Here's how the part is built. I have some questions about the finished solid (model axes, mm). Face numbers are marked on the shaded views. Round coordinates to 2 decimals unless told otherwise and drop trailing zeros. Loops run counter-clockwise (first coordinate to the right, second up) from the corner with the lowest first, then second, coordinate; pieces in that order, holes last. Notation, with made-up numbers: (76, -22.5) - (87, -22.5) arc R22 ccw to (87, 1.5) - close; hole circle Ø5 at (44.5, 53). An arc over 180 degrees is marked (long way). Answer as a JSON object with one key per item and string values. Group by question number.
1) Will these pins go through, and if not, where does the flat tip stop? P1, Ø3, axis at y = -1, z = -29, coming from the -X side; P2, Ø6, axis at x = -4.5, z = -20.5, coming from the -Y side; P3, Ø1.5, axis at x = 4, z = -26, coming from the +Y side.
2) I want a section at B-B, the plane z = -26. Please give me the cut outline in (x, y).
3) If we mould it in two halves opening along Y, with no side actions, what happens to the marked faces 1, 2 and 3? For each: pulls with the +Y half, pulls with the -Y half, needs draft (parallel to the pull), parting line crosses it, or undercut.
4) If I drill on line 1 along Z through (x, y) = (-1.5, 1); line 2 along Z through (x, y) = (-5.25, -0.5); line 3 along Y through (x, z) = (0.5, -23.5), over which ranges is the centre line in solid material (lowest first)? Write a range as [from, to].
5) I want a section at A-A, the plane x = 0. Please give me the cut outline in (y, z), then the cut area to 3 significant figures.
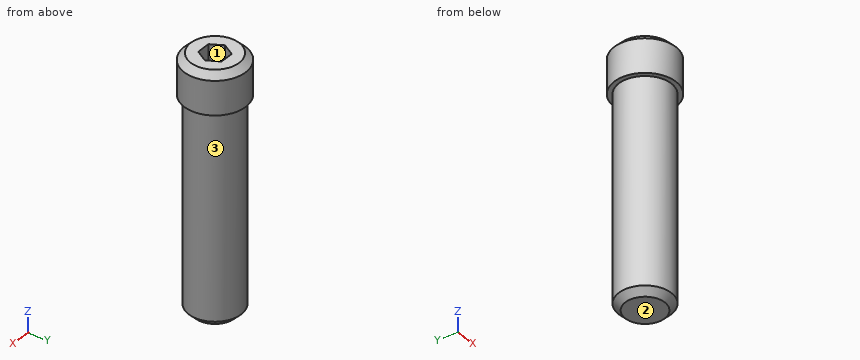
Solid Edge part; units mm, degrees
sketch "Sketch1" plane through (0, 0, 0) normal (0, 0, 1) x (1, 0, 0)
  circle A0 centre (0, 0) radius 7.4549
extrude "Protrusion1" add sketch "Sketch1" along normal blind 9.7282
chamfer "Chamfer_1" distance 1.5875 angle 45 1 edges at (-7.4549, 0, 9.7282)
sketch "Sketch2" plane through (0, 0, 0) normal (0, 0, -1) x (0, -1, 0)
  circle A0 centre (0, 0) radius 6.35
extrude "ExtrudedProtrusion_3" add sketch "Sketch2" along normal blind 50.8
chamfer "Chamfer_2" distance 1.5875 angle 45 1 edges at (0, 6.35, -50.8)
sketch "Sketch3" plane through (0, 0, 9.7282) normal (0, 0, 1) x (0, -1, 0)
  line L0 (0, 3.2856) -> (-2.8454, 1.6428)
  line L1 (-2.8454, 1.6428) -> (-2.8454, -1.6428)
  line L2 (-2.8454, -1.6428) -> (0, -3.2856)
  line L3 (0, -3.2856) -> (2.8454, -1.6428)
  line L4 (2.8454, -1.6428) -> (2.8454, 1.6428)
  line L5 (2.8454, 1.6428) -> (0, 3.2856)
extrude "ExtrudedCutout_1" cut sketch "Sketch3" against normal blind 4.953
properties part number "23415" material "Steel"
Outcome:
{
 "1": {"P1": "x = -6.35", "P2": "y = -6.17", "P3": "y = 5.46"},
 "2": {"outline": "circle Ø12.7 at (0, 0)"},
 "3": {"face 1": "undercut", "face 2": "needs draft", "face 3": "parting line crosses it"},
 "4": {"line 1": "[-50.8, 4.78]", "line 2": "[-50.29, 9.73]", "line 3": "[-6.33, 6.33]"},
 "5": {"outline": "(-7.45, 0) - (-6.35, 0) - (-6.35, -49.21) - (-4.76, -50.8) - (4.76, -50.8) - (6.35, -49.21) - (6.35, 0) - (7.45, 0) - (7.45, 8.14) - (5.87, 9.73) - (2.85, 9.73) - (2.85, 4.78) - (-2.85, 4.78) - (-2.85, 9.73) - (-5.87, 9.73) - (-7.45, 8.14) - close", "area": "757 mm^2"}
}
